Could you check a few things on this model? Use its own coordinates, in mm. Coordinates: 2 decimals unless noted, no trailing zeros. Loops run counter-clockwise (first coordinate to the right, second up) from the corner with the lowest first, then second, coordinate; pieces in that order, holes last. Notation, with made-up numbers: M 2,64 L 12,64 A21 ccw 12,83 Z; hole C -34.5,54 d11. An arc over 180 degrees is marked long. Write each question's results on one line, items separated by ' | '.
```python
from build123d import *

# Parameters (mm, degrees)
SKETCH1_W           = 175
SKETCH1_H           = 63
BOSS_EXTRUDE1_DEPTH = 2.5
SKETCH2_W           = 160
SKETCH2_H           = 40
CUT_EXTRUDE1_DEPTH  = 2.5
SKETCH5_W           = 175
SKETCH5_H           = 45
BOSS_EXTRUDE3_DEPTH = 2.5
BOSS_EXTRUDE2_DEPTH = 108
SKETCH4_R           = 1.65
CUT_EXTRUDE2_DEPTH  = 3.5


with BuildPart() as part:
    # Sketch1 → Boss-Extrude1 (new body)
    with BuildSketch(Plane.XY):
        Rectangle(SKETCH1_W, SKETCH1_H)
    extrude(amount=BOSS_EXTRUDE1_DEPTH)

    # Sketch2 → Cut-Extrude1 (cut)
    with BuildSketch(Plane.XY.offset(2.5)):
        with Locations((0, -2.5)):
            Rectangle(SKETCH2_W, SKETCH2_H)
    extrude(amount=-CUT_EXTRUDE1_DEPTH, mode=Mode.SUBTRACT)

    # Sketch5 → Boss-Extrude3 (add)
    with BuildSketch(Plane.XY.offset(2.5)):
        with Locations((0, 54)):
            Rectangle(SKETCH5_W, SKETCH5_H)
    extrude(amount=-BOSS_EXTRUDE3_DEPTH)

    # Sketch3 → Boss-Extrude2 (add)
    with BuildSketch(Plane(origin=(0, -31.5, 0), x_dir=(1, 0, 0), z_dir=(0, 1, 0))):
        Polygon((-87.5, -2.5), (-103.131306451, -2.5), (-110, 0), (-87.5, 0), align=None)
    boss_extrude2 = extrude(amount=BOSS_EXTRUDE2_DEPTH)

    # Mirror1: Boss-Extrude2 across plane
    add(boss_extrude2.mirror(Plane(origin=(0, 0, 0), x_dir=(0, 0, 1), z_dir=(1, 0, 0))))

    # Sketch4 → Cut-Extrude2 (cut, through all)
    with BuildSketch(Plane(origin=(0, 0, 0), x_dir=(-1, 0, 0), z_dir=(0, 0, -1))):
        with Locations((-32.825, 29)):
            Circle(SKETCH4_R)
    cut_extrude2 = extrude(amount=-CUT_EXTRUDE2_DEPTH, mode=Mode.SUBTRACT)

    # Mirror2: Cut-Extrude2 across plane
    add(cut_extrude2.mirror(Plane(origin=(0, 0, 0), x_dir=(0, 0, 1), z_dir=(1, 0, 0))), mode=Mode.SUBTRACT)


solid = part.part
```
(1) Please list where this line runs through material, in increasing order: probe 1 along Y at (x, z) = (59, 1.45). Write a range as from..to.
Reported:
probe 1: y = -31.5..-22.5, 17.5..76.5
(2) Will these pins go through, and if not, where does the flat tip stop? P1, Ø4.5, axis at x = -32.825, y = 29, coming from the +Z side; P2, Ø2.5, axis at x = 32.825, y = 29, coming from the +Z side.
Reported:
P1: stops at z = 2.5 | P2: passes through
(3) Imagine slicing it at D-D, the plane y = 58. List the corners of the cut face in (x, z) for me, and give its area (3 significant figures).
Reported:
outline: M -110,0 L 110,0 L 103.13,2.5 L -103.13,2.5 Z | area: 533 mm2
(4) Imagine slicing it at A-A, the plane y = -20.5. List the corners of the cut face in (x, z) for me.
Reported:
outline: M -110,0 L -80,0 L -80,2.5 L -103.13,2.5 Z; M 80,0 L 110,0 L 103.13,2.5 L 80,2.5 Z
(5) Imagine slicing it at B-B, the plane x = -65.5. List the corners of the cut face in (y, z) for me, and give its area (3 significant figures).
Reported:
outline: M -31.5,0 L -22.5,0 L -22.5,2.5 L -31.5,2.5 Z; M 17.5,0 L 76.5,0 L 76.5,2.5 L 17.5,2.5 Z | area: 170 mm2
(6) Imagine slicing it at C-C, the plane z = 0.45. List the corners of the cut face in (x, y) for me (3 decimals), and give its area (3 significant figures).
Reported:
outline: M -108.764,-31.5 L 108.764,-31.5 L 108.764,76.5 L -108.764,76.5 Z; hole M -80,-22.5 L 80,-22.5 L 80,17.5 L -80,17.5 Z; hole C -32.825,29 d3.3; hole C 32.825,29 d3.3 | area: 17,100 mm2
